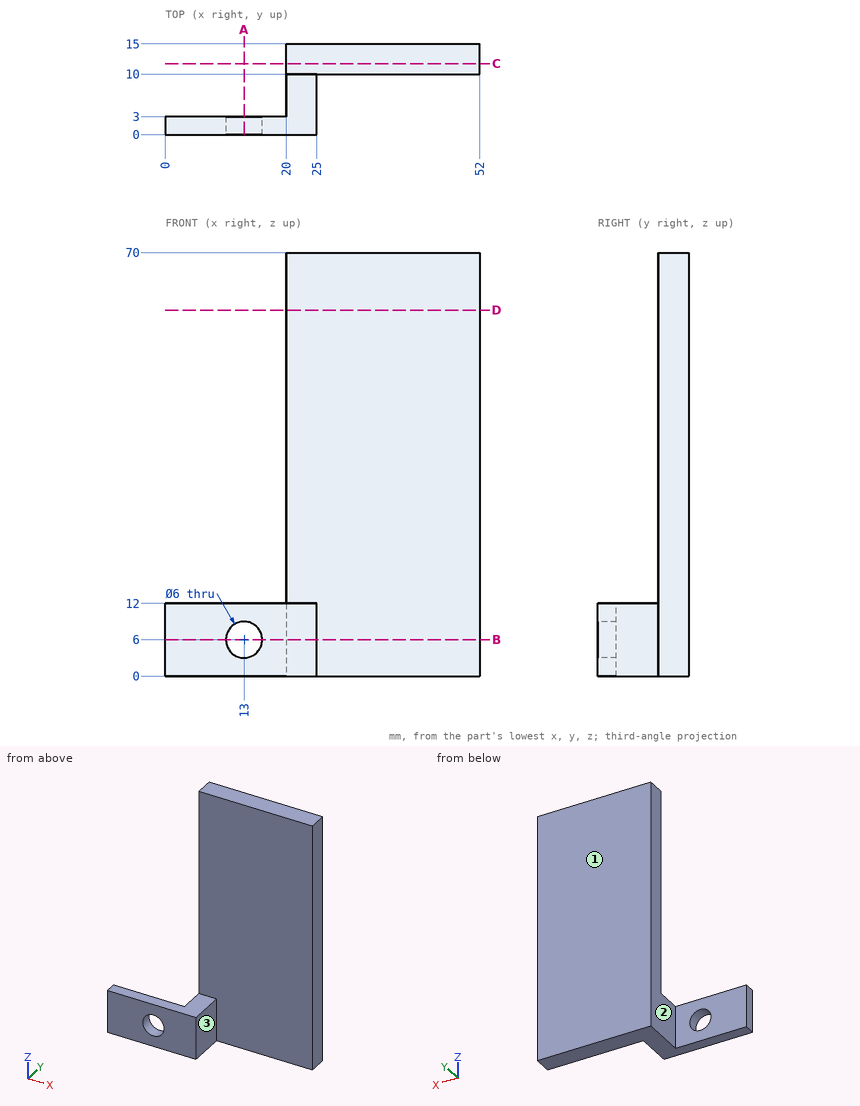
Design review of the part shown in the three views and the two pictorial views. Dimensions are in mm from the part's minimum x, y and z. A direction names the side the tool comes from. Round coordinates to 2 decimals unless told otherwise and drop trailing zeros. Write each loop counter-clockwise with the first axis right and the second up, starting at its lowest first coordinate (ties: lowest second). Pieces come first, ordered by that corner, then holes. Notation, with made-up numbers: (36.25, 60) -> (55.25, 60) arc R27 cw to (55.25, 80) -> close; hole circle Ø1 at (-15, 76.5). An arc over 180 degrees is marked (long way). Write item = value, one per line. Start each with the question number.
1) Clearance check with flat-ended pins moving along their axes: pin 1 (8 mm diameter, centred on y = 10.5, z = 58, fed in from -X); pin 2 (9.5 mm diameter, centred on x = 5, z = 6, fed in from +Y). State where each tip first meets the part, or that it passes through.
2) Take a section at A-A, the plane x = 13. State the section outline as (y, z) points.
3) Take a section at C-C, the plane y = 11.75. State the section outline as (x, z) points, plus the area to 3 significant figures.
4) Take a section at D-D, the plane z = 60.5. State the section outline as (x, y) points, plus the area to 3 significant figures.
5) Wall thickness on probe 1 along Z at (x, y) = (13, 0.8); probe 2 along Y at (x, z) = (44.5, 42); probe 3 along Z at (x, y) = (21, 5): over which ranges is each line inside the solid? List them lowest first. Write a range as from..to.
6) Tool access review of the marked faces 1, 2 and 3: name each direction out of +Z, -Z, +X, -X, +Y, -Y from which nothing blocks a thin tool from reaching the whole face with its end or side.
7) Take a section at B-B, the plane z = 6. State the section outline as (x, y) points.
Results list:
q1.pin_1 = 20
q1.pin_2 = 3
q2.outline = (0, 0) -> (3, 0) -> (3, 3) -> (0, 3) -> close; (0, 9) -> (3, 9) -> (3, 12) -> (0, 12) -> close
q3.outline = (20, 0) -> (52, 0) -> (52, 70) -> (20, 70) -> close
q3.area = 2,240 mm²
q4.outline = (20, 10) -> (52, 10) -> (52, 15) -> (20, 15) -> close
q4.area = 160 mm²
q5.probe_1 = 0..3, 9..12
q5.probe_2 = 10..15
q5.probe_3 = 0..12
q6.face_1 = +Z, -Z, +X, -X, +Y
q6.face_2 = +Z, -Z, -X, +Y
q6.face_3 = +Z, -Z, +X, -Y
q7.outline = (0, 0) -> (10, 0) -> (10, 3) -> (0, 3) -> close; (16, 0) -> (25, 0) -> (25, 10) -> (52, 10) -> (52, 15) -> (20, 15) -> (20, 3) -> (16, 3) -> close
